Geometry: final body of the model. Coordinates: model frame, mm. Face numbers are marked on the shaded views. A direction names the side the tool comes from. Coordinates: 2 decimals unless noted, no trailing zeros. Write each loop counter-clockwise with the first axis right and the second up, starting at its lowest first coordinate (ties: lowest second). Pieces come first, ordered by that corner, then holes. Notation, with made-up numbers: (27.5, -19) -> (59.5, -19) arc R22 ccw to (59.5, 10) -> close; hole circle Ø7 at (23, 78). An arc over 180 degrees is marked (long way). Answer as a JSON object with one key per item and string values. Group by question number.
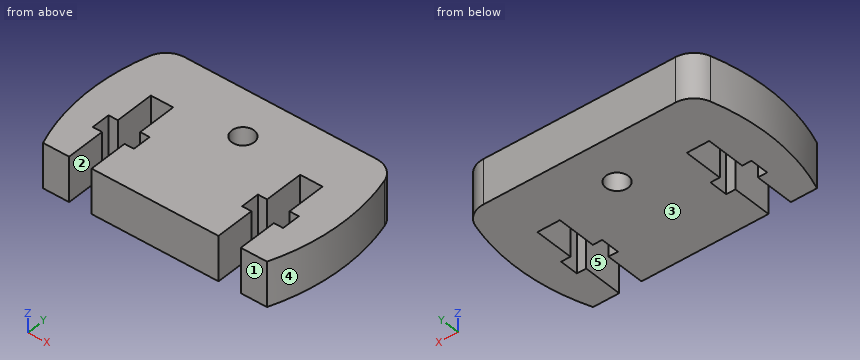
```python
from build123d import *

# Parameters (mm, degrees)
SKETCH_1_R      = 1.5
EXTRUDE_1_DEPTH = 6


with BuildPart() as part:
    # Эскиз1 → Бобышка-Вытянуть1 (new body)
    with BuildSketch(Plane.XY):
        with BuildLine():
            Line((0, 0), (3.5, 0))
            Line((3.5, 0), (3.5, 5.25))
            Line((3.5, 5.25), (2.25, 5.25))
            Line((2.25, 5.25), (2.25, 7.75))
            Line((2.25, 7.75), (3.5, 7.75))
            Line((3.5, 7.75), (3.5, 13))
            Line((3.5, 13), (6.5, 13))
            Line((6.5, 13), (6.5, 7.75))
            Line((6.5, 7.75), (7.75, 7.75))
            Line((7.75, 7.75), (7.75, 5.25))
            Line((7.75, 5.25), (6.5, 5.25))
            Line((6.5, 5.25), (6.5, 0))
            Line((6.5, 0), (23.5, 0))
            Line((23.5, 0), (23.5, 5.25))
            Line((23.5, 5.25), (22.25, 5.25))
            Line((22.25, 5.25), (22.25, 7.75))
            Line((22.25, 7.75), (23.5, 7.75))
            Line((23.5, 7.75), (23.5, 13))
            Line((23.5, 13), (26.5, 13))
            Line((26.5, 13), (26.5, 7.75))
            Line((26.5, 7.75), (27.75, 7.75))
            Line((27.75, 7.75), (27.75, 5.25))
            Line((27.75, 5.25), (26.5, 5.25))
            Line((26.5, 5.25), (26.5, 0))
            Line((26.5, 0), (30, 0))
            ThreePointArc((30, 0), (31.823751247, 8.860593438), (30.726698908, 17.840162517))
            ThreePointArc((30.726698908, 17.840162517), (29.646678597, 19.400050786), (27.846746313, 20))
            Line((27.846746313, 20), (2.153253687, 20))
            ThreePointArc((2.153253687, 20), (0.353321403, 19.400050786), (-0.726698908, 17.840162517))
            ThreePointArc((-0.726698908, 17.840162517), (-1.823751247, 8.860593438), (0, 0))
        make_face()
        with Locations((15, 14)):
            Circle(SKETCH_1_R, mode=Mode.SUBTRACT)
    extrude(amount=EXTRUDE_1_DEPTH)


solid = part.part
```
Item 1: Ray query, L1, parallel to X at y = 10.5, z = 1.1; L2, parallel to Y at x = 15, z = 2.9; L3, parallel to Y at x = 4.5, z = 3.55. Return the intervals inside material, ascending. Write a range as [from, to].
Item 2: Mould query, pull axis X, two halves, no side actions, for the marked faces 3, 4 and 5. Classes: +X half, -X half, draft (parallel to the pull), parting line (faces both ways), or undercut.
Item 3: Section A-A on x = 15. Output: boundary loops of the cut face in (y, z), then the cut area to 3 significant figures.
Item 4: Set-up query: the marked faces 1 and 2. Return all of +Z, -Z, +X, -X, +Y, -Y with unobstructed straight access to the full face (end or side cutting, diameter ignored); none if empty.
Item 5: Section B-B on y = 10. Output: boundary loops of the cut face in (x, z).
Item 6: Contact query for flat-ended pins moving along their axis: pin 1 (3 mm diameter, centred on y = 5.5, z = 4.5, fed in from -X); pin 2 (2.5 mm diameter, centred on y = 3.5, z = 2, fed in from +X); pin 3 (1.2 mm diameter, centred on y = 6, z = 4.5, fed in from -X). Output: stop coordinate, or through.
Item 7: Section D-D on y = 14. Output: boundary loops of the cut face in (x, z), then the cut area to 3 significant figures.
Answer sheet:
{
 "1": {"L1": "x = [-1.84, 3.5], [6.5, 23.5], [26.5, 31.84]", "L2": "y = [0, 12.5], [15.5, 20]", "L3": "y = [13, 20]"},
 "2": {"face 3": "draft", "face 4": "+X half", "face 5": "undercut"},
 "3": {"outline": "(0, 0) -> (12.5, 0) -> (12.5, 6) -> (0, 6) -> close; (15.5, 0) -> (20, 0) -> (20, 6) -> (15.5, 6) -> close", "area": "102 mm^2"},
 "4": {"face 1": "+Z, -Z, +X, -X, -Y", "face 2": "+Z, -Z, -Y"},
 "5": {"outline": "(-1.85, 0) -> (3.5, 0) -> (3.5, 6) -> (-1.85, 6) -> close; (6.5, 0) -> (23.5, 0) -> (23.5, 6) -> (6.5, 6) -> close; (26.5, 0) -> (31.85, 0) -> (31.85, 6) -> (26.5, 6) -> close"},
 "6": {"pin 1": "stops at x = -1.69", "pin 2": "stops at x = 31.35", "pin 3": "stops at x = -1.64"},
 "7": {"outline": "(-1.56, 0) -> (13.5, 0) -> (13.5, 6) -> (-1.56, 6) -> close; (16.5, 0) -> (31.56, 0) -> (31.56, 6) -> (16.5, 6) -> close", "area": "181 mm^2"}
}
